```python
from build123d import *

# Parameters (mm, degrees)
SKETCH1_W           = 170
SKETCH1_H           = 61
BOSS_EXTRUDE1_DEPTH = 2
SKETCH2_W           = 170
SKETCH2_H           = 2
BOSS_EXTRUDE2_DEPTH = 17
SKETCH3_W           = 166
SKETCH3_H           = 2
BOSS_EXTRUDE3_DEPTH = 17
SKETCH4_W           = 70
SKETCH4_H           = 2
BOSS_EXTRUDE4_DEPTH = 42
SKETCH5_W           = 4
SKETCH5_H           = 8
CUT_EXTRUDE1_DEPTH  = 39
FILLET1_R           = 2
SKETCH6_W           = 2
SKETCH6_H           = 42
BOSS_EXTRUDE5_DEPTH = 17
SKETCH9_W           = 66
SKETCH9_H           = 2
BOSS_EXTRUDE6_DEPTH = 17
SKETCH10_W          = 6
SKETCH10_H          = 3
CUT_EXTRUDE2_DEPTH  = 10
SKETCH11_W          = 6
SKETCH11_H          = 3
CUT_EXTRUDE3_DEPTH  = 10
SKETCH12_W          = 6
SKETCH12_H          = 3
CUT_EXTRUDE4_DEPTH  = 10
SKETCH13_W          = 6
SKETCH13_H          = 3
CUT_EXTRUDE5_DEPTH  = 10
CUT_EXTRUDE6_DEPTH  = 2
SKETCH15_W          = 66
SKETCH15_H          = 40
SKETCH15_W_2        = 166
SKETCH15_H_2        = 57
BOSS_EXTRUDE7_DEPTH = 13
BOSS_EXTRUDE8_DEPTH = 2
SKETCH17_W          = 14
SKETCH17_H          = 8.1
CUT_EXTRUDE7_DEPTH  = 2
FILLET2_R           = 1
FILLET3_R           = 1


with BuildPart() as part:
    # Sketch1 → Boss-Extrude1 (new body)
    with BuildSketch(Plane(origin=(0, 0, 0), x_dir=(1, 0, 0), z_dir=(0, 1, 0))):
        with Locations((85, -30.5)):
            Rectangle(SKETCH1_W, SKETCH1_H)
    extrude(amount=BOSS_EXTRUDE1_DEPTH)

    # Sketch2 → Boss-Extrude2 (add)
    with BuildSketch(Plane(origin=(0, 2, 0), x_dir=(1, 0, 0), z_dir=(0, 1, 0))):
        with Locations((85, -1)):
            Rectangle(SKETCH2_W, SKETCH2_H)
    extrude(amount=BOSS_EXTRUDE2_DEPTH)

    # Sketch3 → Boss-Extrude3 (add)
    with BuildSketch(Plane(origin=(0, 2, 0), x_dir=(1, 0, 0), z_dir=(0, 1, 0))):
        Polygon((0, -2), (0, -61), (2, -61), (2, -59), (2, -2), align=None)
        Polygon((168, -59), (168, -61), (170, -61), (170, -2), (168, -2), align=None)
        with Locations((85, -60)):
            Rectangle(SKETCH3_W, SKETCH3_H)
    extrude(amount=BOSS_EXTRUDE3_DEPTH)

    # Sketch4 → Boss-Extrude4 (add)
    with BuildSketch(Plane(origin=(0, 0, 0), x_dir=(-1, 0, 0), z_dir=(0, 0, -1))):
        with Locations((-85, 1)):
            Rectangle(SKETCH4_W, SKETCH4_H)
    extrude(amount=BOSS_EXTRUDE4_DEPTH)

    # Sketch5 → Cut-Extrude1 (cut)
    with BuildSketch(Plane(origin=(0, 0, 0), x_dir=(-1, 0, 0), z_dir=(0, 0, -1))):
        with Locations((-55.116937283, 19)):
            Rectangle(SKETCH5_W, SKETCH5_H)
    extrude(amount=-CUT_EXTRUDE1_DEPTH, mode=Mode.SUBTRACT)

    # Fillet1
    fillet1_edges = [part.edges().sort_by_distance(p)[0] for p in [
        (53.116937283, 19, 1),
        (57.116937283, 19, 1),
    ]]
    fillet(fillet1_edges, radius=FILLET1_R)

    # Sketch6 → Boss-Extrude5 (add)
    with BuildSketch(Plane(origin=(0, 2, 0), x_dir=(1, 0, 0), z_dir=(0, 1, 0))):
        with Locations((119, 21)):
            Rectangle(SKETCH6_W, SKETCH6_H)
    extrude(amount=BOSS_EXTRUDE5_DEPTH)

    # Sketch9 → Boss-Extrude6 (add)
    with BuildSketch(Plane(origin=(0, 2, 0), x_dir=(1, 0, 0), z_dir=(0, 1, 0))):
        Polygon((52, 42), (50, 42), (50, 0), (52, 0), (52, 40), align=None)
        with Locations((85, 41)):
            Rectangle(SKETCH9_W, SKETCH9_H)
    extrude(amount=BOSS_EXTRUDE6_DEPTH)

    # Sketch10 → Cut-Extrude2 (cut)
    with BuildSketch(Plane.XY.offset(61)):
        with Locations((43, 15.5)):
            Rectangle(SKETCH10_W, SKETCH10_H)
        with Locations((127, 15.5)):
            Rectangle(SKETCH10_W, SKETCH10_H)
    extrude(amount=-CUT_EXTRUDE2_DEPTH, mode=Mode.SUBTRACT)

    # Sketch11 → Cut-Extrude3 (cut)
    with BuildSketch(Plane.ZY):
        with Locations((30.5, 15.5)):
            Rectangle(SKETCH11_W, SKETCH11_H)
    extrude(amount=-CUT_EXTRUDE3_DEPTH, mode=Mode.SUBTRACT)

    # Sketch12 → Cut-Extrude4 (cut)
    with BuildSketch(Plane(origin=(0, 0, -42), x_dir=(-1, 0, 0), z_dir=(0, 0, -1))):
        with Locations((-85, 15.5)):
            Rectangle(SKETCH12_W, SKETCH12_H)
    extrude(amount=-CUT_EXTRUDE4_DEPTH, mode=Mode.SUBTRACT)

    # Sketch13 → Cut-Extrude5 (cut)
    with BuildSketch(Plane(origin=(170, 0, 0), x_dir=(0, 0, -1), z_dir=(1, 0, 0))):
        with Locations((-30.5, 15.5)):
            Rectangle(SKETCH13_W, SKETCH13_H)
    extrude(amount=-CUT_EXTRUDE5_DEPTH, mode=Mode.SUBTRACT)

    # Sketch14 → Cut-Extrude6 (cut)
    with BuildSketch(Plane.XZ):
        Polygon((0, 61), (0, 0), (50, 0), (50, -42), (120, -42), (120, 0), (170, 0), (170, 61), align=None)
    extrude(amount=-CUT_EXTRUDE6_DEPTH, mode=Mode.SUBTRACT)

    # Sketch15 → Boss-Extrude7 (add)
    with BuildSketch(Plane.XZ.offset(-2)):
        Polygon((170, 61), (0, 61), (0, 0), (50, 0), (50, -42), (120, -42), (120, 0), (170, 0), align=None)
        with Locations((85, -20)):
            Rectangle(SKETCH15_W, SKETCH15_H, mode=Mode.SUBTRACT)
        with Locations((85, 30.5)):
            Rectangle(SKETCH15_W_2, SKETCH15_H_2, mode=Mode.SUBTRACT)
    extrude(amount=BOSS_EXTRUDE7_DEPTH)

    # Sketch16 → Boss-Extrude8 (add)
    with BuildSketch(Plane.XZ.offset(11)):
        Polygon((120, -42), (120, 0), (170, 0), (170, 61), (0, 61), (0, 0), (50, 0), (50, -42), align=None)
    extrude(amount=BOSS_EXTRUDE8_DEPTH)

    # Sketch17 → Cut-Extrude7 (cut)
    with BuildSketch(Plane.ZY):
        with Locations((30.5, 6.05)):
            Rectangle(SKETCH17_W, SKETCH17_H)
    extrude(amount=-CUT_EXTRUDE7_DEPTH, mode=Mode.SUBTRACT)

    # Fillet2
    fillet2_edges = [part.edges().sort_by_distance(p)[0] for p in [
        (50, 3, -42),
        (120, 3, -42),
        (120, 3, 0),
        (50, 3, 0),
        (0, 3, 0),
        (170, 3, 0),
        (170, 3, 61),
        (0, 3, 61),
    ]]
    fillet(fillet2_edges, radius=FILLET2_R)

    # Fillet3
    fillet3_edges = [part.edges().sort_by_distance(p)[0] for p in [
        (1, 2, 23.5),
        (1, 10.1, 23.5),
        (1, 10.1, 37.5),
        (1, 2, 37.5),
    ]]
    fillet(fillet3_edges, radius=FILLET3_R)


solid = part.part
```
Work out the finished part from the listing and answer in its coordinate system (mm). A direction names the side the tool comes from. Coordinates: 2 decimals unless noted, no trailing zeros. Write each loop counter-clockwise with the first axis right and the second up, starting at its lowest first coordinate (ties: lowest second). Pieces come first, ordered by that corner, then holes.
Q1. A cutting plane is placed at C-C, the plane z = 40. Give the vertices of the cut face in (x, y).
Q2. Determine the mould class of faces 5 (the face through (84, -13, 22)), 6 (the face through (84, -11, 31)), 7 (the face through (170, 3, 30)) for opening direction X: released by +X, released by -X, zero draft, split by the parting line, or undercut.
Q3. Find the intervals of material crossed by line 1 (Z direction, x = 114.5, y = 1.5); line 2 (Z direction, x = 8.5, y = 8.5); line 3 (X direction, y = 5.5, z = 9.5), in increasing order.
Q4. A cutting plane is placed at D-D, the plane x = 95. Give the vertices of the cut face in (y, z).
Q5. A cutting plane is placed at B-B, the plane y = 7. Give the vertices of the cut face in (x, z), then the cut area to 3 significant figures.
Q6. Each of these flat-tipped pins is pushed along its axis until it touches: pin 1 Ø4 at (x, z) = (78.5, 14) entering from +Y; pin 2 Ø8 at (y, z) = (-8.5, -7.5) entering from +X; pin 3 Ø0.6 at (y, z) = (16, 0.5) entering from +X. Where does it stop, or does it pass through?
Q7. A cutting plane is placed at A-A, the plane y = -6. Give the vertices of the cut face in (x, z).
Q8. Which of the six approach directions +Z, -Z, +X, -X, +Y, -Y give full straight-line access (tool end or side, diameter ignored) to faces 1 (the face through (85, 4, -40)), 2 (the face through (25, 3, 0)), 3 (the face through (85, 3, -42)), 4 (the face through (120, 3, -21))?
Findings below:
1. outline: (0, -13) - (170, -13) - (170, 19) - (168, 19) - (168, -11) - (2, -11) - (2, 19) - (0, 19) - close
2. face 5: zero draft
2. face 6: undercut
2. face 7: released by +X
3. line 1: z = -42 to -40, 0 to 2, 59 to 61
3. line 2: z = 0 to 2, 59 to 61
3. line 3: x = 0 to 2, 168 to 170
4. outline: (-13, -42) - (19, -42) - (19, -40) - (-11, -40) - (-11, 0) - (19, 0) - (19, 2) - (-11, 2) - (-11, 59) - (19, 59) - (19, 61) - (-13, 61) - close
5. outline: (0, 1) arc R1 ccw to (1, 0) - (49, 0) arc R1 cw to (50, -1) - (50, -41) arc R1 ccw to (51, -42) - (119, -42) arc R1 ccw to (120, -41) - (120, -1) arc R1 cw to (121, 0) - (169, 0) arc R1 ccw to (170, 1) - (170, 60) arc R1 ccw to (169, 61) - (1, 61) arc R1 ccw to (0, 60) - (0, 37.5) - (2, 37.5) - (2, 59) - (168, 59) - (168, 2) - (2, 2) - (2, 23.5) - (0, 23.5) - close; hole (52, -40) - (118, -40) - (118, 0) - (52, 0) - close
5. area: 1,180 mm2
6. pin 1: stops at y = -11
6. pin 2: stops at x = 120
6. pin 3: stops at x = 169.98
7. outline: (0, 1) arc R1 ccw to (1, 0) - (49, 0) arc R1 cw to (50, -1) - (50, -41) arc R1 ccw to (51, -42) - (119, -42) arc R1 ccw to (120, -41) - (120, -1) arc R1 cw to (121, 0) - (169, 0) arc R1 ccw to (170, 1) - (170, 60) arc R1 ccw to (169, 61) - (1, 61) arc R1 ccw to (0, 60) - close; hole (2, 2) - (168, 2) - (168, 59) - (2, 59) - close; hole (52, -40) - (118, -40) - (118, 0) - (52, 0) - close
8. face 1: +Y
8. face 2: -Z, -X, +Y, -Y
8. face 3: -Z, +X, -X, +Y, -Y
8. face 4: -Z, +X, +Y, -Y
